The figure shows three views and two pictorial views of one solid part (mm, origin at its lowest corner). Answer the questions. A direction names the side the tool comes from. Round coordinates to 2 decimals unless told otherwise and drop trailing zeros. Write each loop counter-clockwise with the first axis right and the second up, starting at its lowest first coordinate (ties: lowest second). Pieces come first, ordered by that corner, then holes. Notation, with made-up numbers: M -28,-28.75 L 8,-28.75 A26 cw 8,10.25 Z; hole C 67,28 d2. An arc over 180 degrees is marked long. Answer in a Markdown table with one row per item.
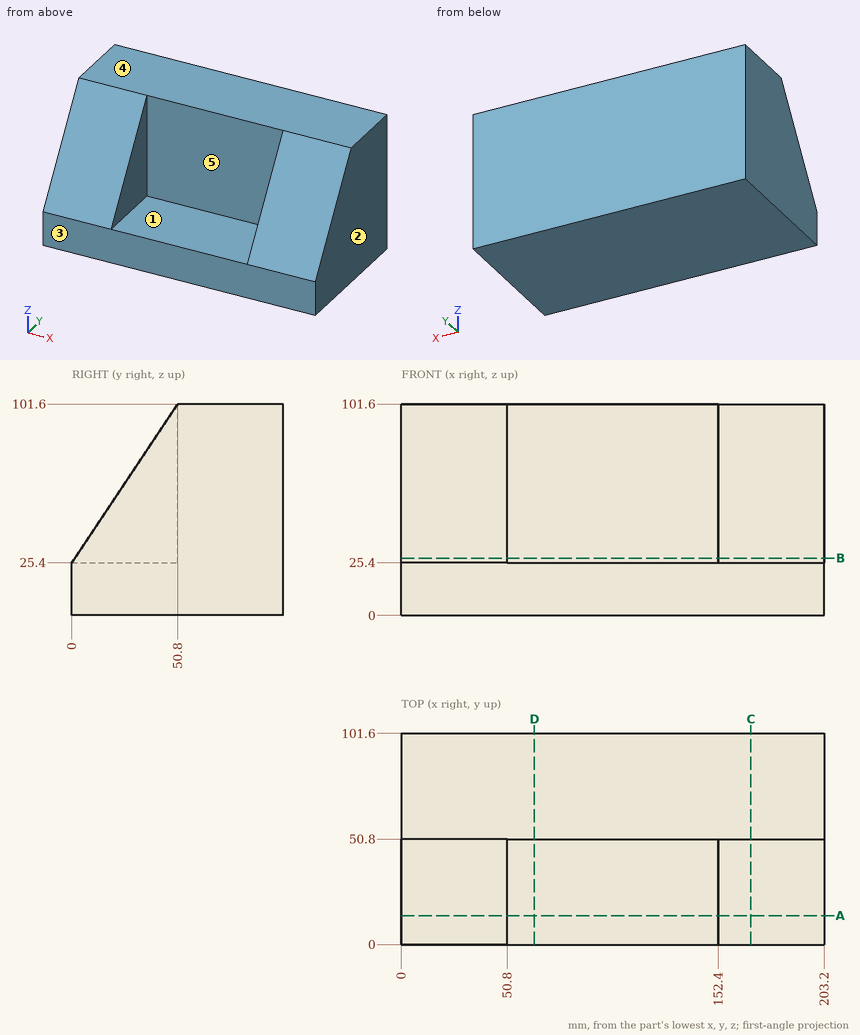
1. The part is cut by section A-A (y = 14). Determine the outline of the cut face in (x, z), plus the area to 3 significant figures.
Calculated:
| item | result |
|---|---|
| outline | M 0,0 L 203.2,0 L 203.2,46.4 L 152.4,46.4 L 152.4,25.4 L 50.8,25.4 L 50.8,46.4 L 0,46.4 Z |
| area | 7,290 mm² |
2. The part is cut by section D-D (x = 64). Determine the outline of the cut face in (y, z).
Calculated:
| item | result |
|---|---|
| outline | M 0,0 L 101.6,0 L 101.6,101.6 L 50.8,101.6 L 50.8,25.4 L 0,25.4 Z |
3. A tool of negligible diameter and unlimited length cuts with its end or side. For the marked faces 4 and 5, from which of +Z, -Z, +X, -X, +Y, -Y can it reach the whole face along a straight path? Write none if from no direction.
Calculated:
| item | result |
|---|---|
| face 4 | +Z, +X, -X, +Y, -Y |
| face 5 | +Z, -Y |
4. The part is cut by section B-B (z = 27.5). Determine the outline of the cut face in (x, y).
Calculated:
| item | result |
|---|---|
| outline | M 0,1.4 L 50.8,1.4 L 50.8,50.8 L 152.4,50.8 L 152.4,1.4 L 203.2,1.4 L 203.2,101.6 L 0,101.6 Z |
5. Given pin 1 (23 mm diameter, centred on x = 84, z = 66, fed in from -Y); pin 2 (3 mm diameter, centred on x = 53, y = 44, fed in from +Z), each flat-ended and moving along its own axis, determine where each tip first touches the part or whether it passes through.
Calculated:
| item | result |
|---|---|
| pin 1 | stops at y = 50.8 |
| pin 2 | stops at z = 25.4 |
6. The part is cut by section C-C (x = 168). Determine the outline of the cut face in (y, z).
Calculated:
| item | result |
|---|---|
| outline | M 0,0 L 101.6,0 L 101.6,101.6 L 50.8,101.6 L 0,25.4 Z |
7. Determine the mould class of the marked faces 1, 2 and 3 for opening direction X: released by +X, released by -X, zero draft, split by the parting line, or undercut.
Calculated:
| item | result |
|---|---|
| face 1 | undercut |
| face 2 | released by +X |
| face 3 | zero draft |
8. Consider line 1 along X through (y, z) = (38, 49); line 2 along Z through (x, y) = (78, 37.5); line 3 along Y through (x, z) = (58.5, 28.5). Determine where each line is inside the solid, lowest interval first. Write a range as from..to.
Calculated:
| item | result |
|---|---|
| line 1 | x = 0..50.8, 152.4..203.2 |
| line 2 | z = 0..25.4 |
| line 3 | y = 50.8..101.6 |
